Can you work these out from the drawing? Everything is in mm from the part's minimum corner. A direction names the side the tool comes from. Give positions to 0.01 mm unless a question says otherwise; leave off trailing zeros. Loops run counter-clockwise (first coordinate to the right, second up) from the corner with the lowest first, then second, coordinate; pieces in that order, holes last. Notation, with made-up numbers: (44, 43) - (91, 43) arc R16 ccw to (91, 65) - close; hole circle Ø10 at (-3.75, 65). An arc over 180 degrees is marked (long way). Answer in a Markdown table with one row per item.
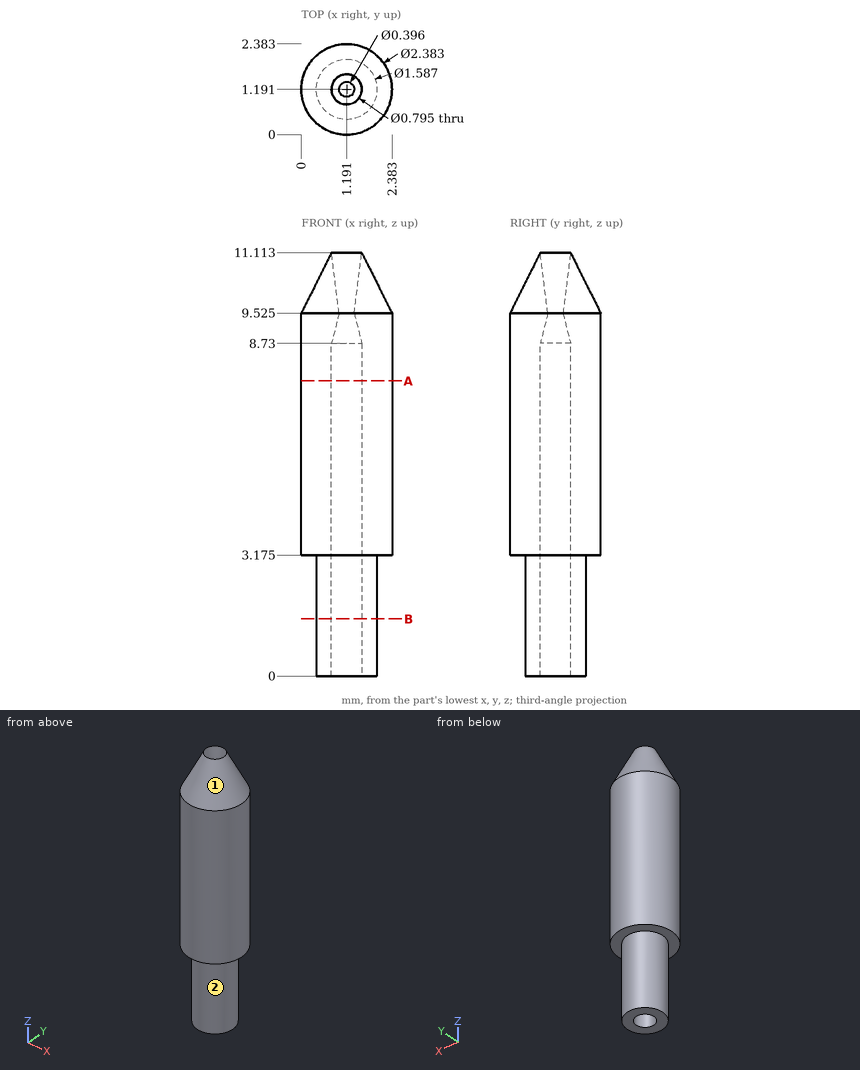
Q1. On a 3-axis mill with a long thin cutter (end or side, diameter ignored), from which of +Z, -Z, +X, -X, +Y, -Y can I reach the whole of each face in a straight line? I mean the marked faces 1 and 2. Say none if no direction works.
Checked values:
| item | result |
|---|---|
| face 1 | +Z |
| face 2 | -Z |
Q2. Imagine slicing it at B-B, the plane z = 1.5. Write out the boundary of the cut face in (x, y) (1 decimal).
Checked values:
| item | result |
|---|---|
| outline | circle Ø1.6 at (1.2, 1.2); hole circle Ø0.8 at (1.2, 1.2) |
Q3. If I drill on line 1 (X direction, y = 1, z = 2.75) (1 decimal); line 2 (X direction, y = 1.15, z = 0.75) (1 decimal); line 3 (Y direction, x = 0.9, z = 8.5) (1 decimal), over which ranges is the centre line in solid material (lowest first)? Write a range as [from, to].
Checked values:
| item | result |
|---|---|
| line 1 | x = [0.4, 0.8], [1.5, 2] |
| line 2 | x = [0.4, 0.8], [1.6, 2] |
| line 3 | y = [0, 0.9], [1.5, 2.3] |
Q4. Imagine slicing it at A-A, the plane z = 7.75. Write out the boundary of the cut face in (x, y) (1 decimal).
Checked values:
| item | result |
|---|---|
| outline | circle Ø2.4 at (1.2, 1.2); hole circle Ø0.8 at (1.2, 1.2) |
